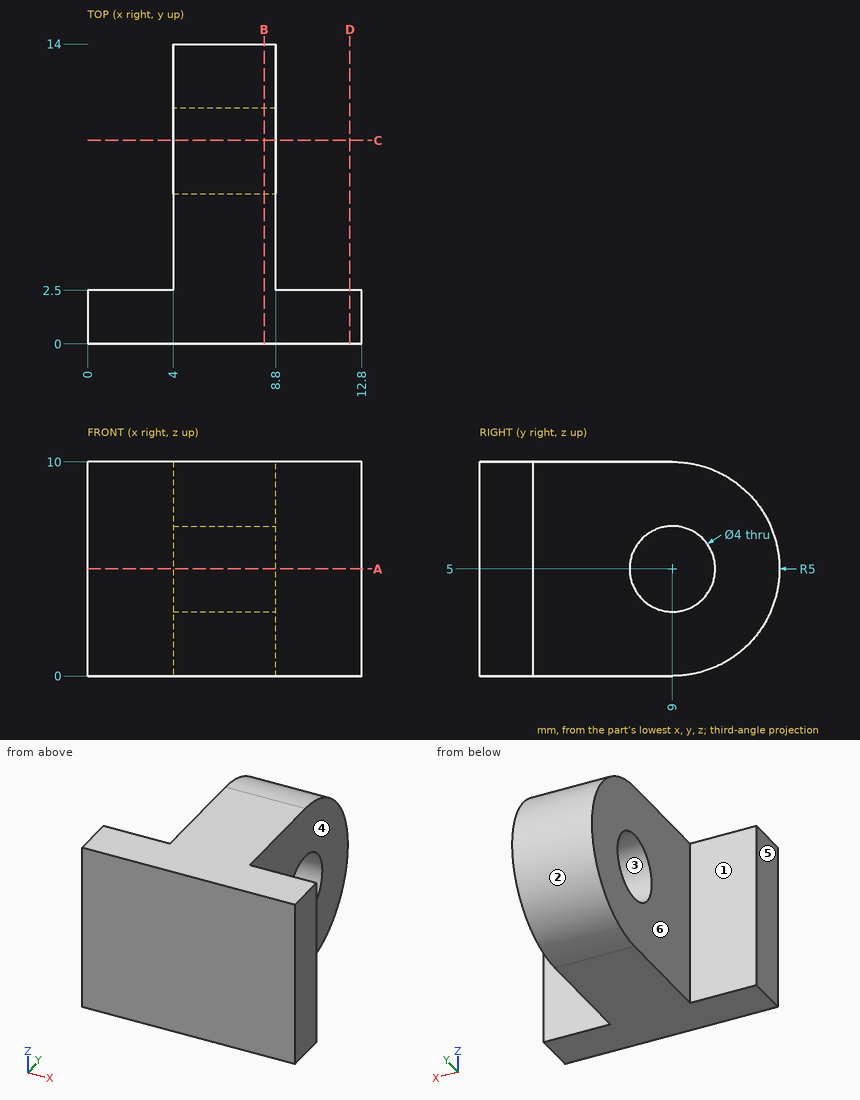
Could you check a few things on this drawing? It's one solid part, dimensions in mm from its lowest x, y, z. A direction names the side the tool comes from. Give positions to 0.01 mm unless a question says otherwise; leave off trailing zeros. Loops run counter-clockwise (first coordinate to the right, second up) from the corner with the lowest first, then second, coordinate; pieces in that order, holes last. Notation, with made-up numbers: (-11.75, 71) -> (23.25, 71) arc R26 ccw to (23.25, 97) -> close; hole circle Ø10 at (51, 42.25). An arc over 180 degrees is marked (long way). Use one line per item in the form item = value. Start each with the question number.
1) Imagine slicing it at D-D (x = 12.25). Please give me the cut outline in (y, z).
2) Thinking about a two-plate mould opening in Z: for the marked faces 1, 2 and 3, which applies, +Z half, -Z half, draft (parallel to the pull), parting line (faces both ways), or undercut?
3) Please list where these lines run through material, in increasing order: line 1 along Z through (x, y) = (7.5, 9); line 2 along X through (y, z) = (9.5, 7.5); line 3 along Y through (x, z) = (12.25, 8).
4) Which directions (+Z, -Z, +X, -X, +Y, -Y) give clear straight access to the entire face, cutting with the end or side of a thin tool? Please do the marked faces 4, 5 and 6.
5) Imagine slicing it at B-B (x = 8.25). Please give me the cut outline in (y, z), then the cut area to 3 significant figures.
6) Imagine slicing it at A-A (z = 5). Please give me the cut outline in (x, y).
7) For P1, Ø3, axis at x = 10.5, z = 3.5, coming from the +Y side; P2, Ø1.5, axis at x = 7.5, y = 11.5, coming from the +Z side; P3, Ø6, axis at y = 9.5, z = 5.5, coming from the -X side; P4, Ø3, axis at y = 9, z = 5, coming from the +X side, each with a flat end and sliding along its axis, tell me the tip position at first contact or that it passes through.
8) Imagine slicing it at C-C (y = 9.5). Please give me the cut outline in (x, z).
Check values:
q1.outline = (0, 0) -> (2.5, 0) -> (2.5, 10) -> (0, 10) -> close
q2.face_1 = draft
q2.face_2 = parting line
q2.face_3 = undercut
q3.line_1 = 0 to 3, 7 to 10
q3.line_2 = 4 to 8.8
q3.line_3 = 0 to 2.5
q4.face_4 = +Z, -Z, +X, +Y
q4.face_5 = +Z, -Z, -X, +Y, -Y
q4.face_6 = +Z, -Z, -X, +Y
q5.outline = (0, 0) -> (9, 0) arc R5 ccw to (9, 10) -> (0, 10) -> close; hole circle Ø4 at (9, 5)
q5.area = 117 mm^2
q6.outline = (0, 0) -> (12.8, 0) -> (12.8, 2.5) -> (8.8, 2.5) -> (8.8, 7) -> (4, 7) -> (4, 2.5) -> (0, 2.5) -> close; (4, 11) -> (8.8, 11) -> (8.8, 14) -> (4, 14) -> close
q7.P1 = 2.5
q7.P2 = 9.68
q7.P3 = 4
q7.P4 = through
q8.outline = (4, 0.03) -> (8.8, 0.03) -> (8.8, 3.06) -> (4, 3.06) -> close; (4, 6.94) -> (8.8, 6.94) -> (8.8, 9.97) -> (4, 9.97) -> close
